```python
from build123d import *

# Parameters (mm, degrees)
BOX085026_W          = 9
BOX085026_H          = 1
BOX085026_DEPTH      = 3.85
FILLET005011017017_R = 0.49
BOX085027_W          = 9
BOX085027_H          = 1
BOX085027_DEPTH      = 3.85
FILLET005011017018_R = 0.49
BOX085028_W          = 9
BOX085028_H          = 1
BOX085028_DEPTH      = 3.85
FILLET005011017019_R = 0.49
BOX085029_W          = 9
BOX085029_H          = 1
BOX085029_DEPTH      = 3.85
FILLET005011017020_R = 0.49
BOX085030_W          = 9
BOX085030_H          = 1
BOX085030_DEPTH      = 3.85
FILLET005011017021_R = 0.49
BOX085025_W          = 9
BOX085025_H          = 9
BOX085025_DEPTH      = 1.7


with BuildPart() as fillet005011017017:
    # Box085026 → Box085026 (new body)
    with BuildSketch(Plane(origin=(25.897, 21.115, 10), x_dir=(1, 0, 0), z_dir=(0, 0, 1))):
        with Locations((4.5, 0.5)):
            Rectangle(BOX085026_W, BOX085026_H)
    extrude(amount=BOX085026_DEPTH)

    # Fillet005011017017
    fillet005011017017_edges = [fillet005011017017.edges().sort_by_distance(p)[0] for p in [
        (30.397, 21.115, 13.85),
        (30.397, 22.115, 13.85),
    ]]
    fillet(fillet005011017017_edges, radius=FILLET005011017017_R)


with BuildPart() as fillet005011017018:
    # Box085027 → Box085027 (new body)
    with BuildSketch(Plane(origin=(25.897, 21.115, 10), x_dir=(1, 0, 0), z_dir=(0, 0, 1))):
        with Locations((4.5, 0.5)):
            Rectangle(BOX085027_W, BOX085027_H)
    extrude(amount=BOX085027_DEPTH)

    # Fillet005011017018
    fillet005011017018_edges = [fillet005011017018.edges().sort_by_distance(p)[0] for p in [
        (30.397, 21.115, 13.85),
        (30.397, 22.115, 13.85),
    ]]
    fillet(fillet005011017018_edges, radius=FILLET005011017018_R)


with BuildPart() as fillet005011017018_1:
    # Fillet005011017018 placement: moved
    add(fillet005011017018.part.moved(Location((0, 2, 0))))


with BuildPart() as fillet005011017019:
    # Box085028 → Box085028 (new body)
    with BuildSketch(Plane(origin=(25.897, 21.115, 10), x_dir=(1, 0, 0), z_dir=(0, 0, 1))):
        with Locations((4.5, 0.5)):
            Rectangle(BOX085028_W, BOX085028_H)
    extrude(amount=BOX085028_DEPTH)

    # Fillet005011017019
    fillet005011017019_edges = [fillet005011017019.edges().sort_by_distance(p)[0] for p in [
        (30.397, 21.115, 13.85),
        (30.397, 22.115, 13.85),
    ]]
    fillet(fillet005011017019_edges, radius=FILLET005011017019_R)


with BuildPart() as fillet005011017019_1:
    # Fillet005011017019 placement: moved
    add(fillet005011017019.part.moved(Location((0, 4, 0))))


with BuildPart() as fillet005011017020:
    # Box085029 → Box085029 (new body)
    with BuildSketch(Plane(origin=(25.897, 21.115, 10), x_dir=(1, 0, 0), z_dir=(0, 0, 1))):
        with Locations((4.5, 0.5)):
            Rectangle(BOX085029_W, BOX085029_H)
    extrude(amount=BOX085029_DEPTH)

    # Fillet005011017020
    fillet005011017020_edges = [fillet005011017020.edges().sort_by_distance(p)[0] for p in [
        (30.397, 21.115, 13.85),
        (30.397, 22.115, 13.85),
    ]]
    fillet(fillet005011017020_edges, radius=FILLET005011017020_R)


with BuildPart() as fillet005011017020_1:
    # Fillet005011017020 placement: moved
    add(fillet005011017020.part.moved(Location((0, 6, 0))))


with BuildPart() as fillet005011017021:
    # Box085030 → Box085030 (new body)
    with BuildSketch(Plane(origin=(25.897, 21.115, 10), x_dir=(1, 0, 0), z_dir=(0, 0, 1))):
        with Locations((4.5, 0.5)):
            Rectangle(BOX085030_W, BOX085030_H)
    extrude(amount=BOX085030_DEPTH)

    # Fillet005011017021
    fillet005011017021_edges = [fillet005011017021.edges().sort_by_distance(p)[0] for p in [
        (30.397, 21.115, 13.85),
        (30.397, 22.115, 13.85),
    ]]
    fillet(fillet005011017021_edges, radius=FILLET005011017021_R)


with BuildPart() as fillet005011017021_1:
    # Fillet005011017021 placement: moved
    add(fillet005011017021.part.moved(Location((0, 8, 0))))


with BuildPart() as obj1:
    # Box085025 → Box085025 (new body)
    with BuildSketch(Plane(origin=(25.897, 21.115, 8.3), x_dir=(1, 0, 0), z_dir=(0, 0, 1))):
        with Locations((4.5, 4.5)):
            Rectangle(BOX085025_W, BOX085025_H)
    extrude(amount=BOX085025_DEPTH)

    # Fusion004008002002002001007002002014: union Fillet005011017017, Fillet005011017018, Fillet005011017019, Fillet005011017020, Fillet005011017021
    add(fillet005011017017.part)
    add(fillet005011017018_1.part)
    add(fillet005011017019_1.part)
    add(fillet005011017020_1.part)
    add(fillet005011017021_1.part)


with BuildPart() as obj1_1:
    # Fusion004008002002002001007002002014 placement: moved
    add(obj1.part.moved(Location((0, 0, -1))))


solid = obj1_1.part
```
Geometry check sheet. Reference: the model listing, model coordinates, mm. A direction names the side the tool comes from. Give positions to 0.01 mm unless a question says otherwise; leave off trailing zeros. Loops run counter-clockwise (first coordinate to the right, second up) from the corner with the lowest first, then second, coordinate; pieces in that order, holes last. Notation, with made-up numbers: M 4,-3.5 L 58,-3.5 A17 ccw 58,2.5 Z; hole C 9,-24 d10. An arc over 180 degrees is marked long. Write item = value, one per line. Start each with the question number.
1. Draft check along Y on faces 3 (the face through (30.3, 24.6, 9)), 4 (the face through (34.897, 25.6, 9.4)), 5 (the face through (30, 21.115, 10)). Enter one of: +Y half, -Y half, draft (parallel to the pull), parting line (faces both ways), or undercut.
2. Section check C-C, the plane y = 29.25. Enter the section's corners in (x, z).
3. Section check A-A, the plane z = 10. Enter the section's corners in (x, y) (3 decimals), plus the area to 3 significant figures.
4. Go/stop test with flat-tipped pins: P1, Ø0.5, axis at x = 32.5, y = 29, coming from the +Z side; P2, Ø1.1, axis at x = 28.5, y = 27, coming from the +Z side; P3, Ø0.5, axis at x = 31.5, y = 24.5, coming from the +Z side. Record where each tip stops, or that it passes through.
5. Section check D-D, the plane y = 26. Enter the section's corners in (x, z).
6. Thickness scan on probe 1 along Y at (x, z) = (26.75, 9.9) (3 decimals); probe 2 along Y at (x, z) = (29.25, 12.65); probe 3 along Z at (x, y) = (31.25, 27). Record the ranges inside material, lowest first.
7. Tool access check on faces 1 (the face through (30, 24.115, 11)), 2 (the face through (25.897, 25.6, 9.4)). Record the directions out of +Z, -Z, +X, -X, +Y, -Y that give a thin tool (end or side, any length) a straight path to the whole face; none if there is none.
Values follow:
q1.face_3 = undercut
q1.face_4 = draft
q1.face_5 = -Y half
q2.outline = M 25.9,7.3 L 34.9,7.3 L 34.9,12.7 L 25.9,12.7 Z
q3.outline = M 25.897,21.115 L 34.897,21.115 L 34.897,22.115 L 25.897,22.115 Z; M 25.897,23.115 L 34.897,23.115 L 34.897,24.115 L 25.897,24.115 Z; M 25.897,25.115 L 34.897,25.115 L 34.897,26.115 L 25.897,26.115 Z; M 25.897,27.115 L 34.897,27.115 L 34.897,28.115 L 25.897,28.115 Z; M 25.897,29.115 L 34.897,29.115 L 34.897,30.115 L 25.897,30.115 Z
q3.area = 45.0 mm^2
q4.P1 = 12.7
q4.P2 = 12.85
q4.P3 = 9
q5.outline = M 25.9,7.3 L 34.9,7.3 L 34.9,12.68 L 25.9,12.68 Z
q6.probe_1 = 21.115 to 22.115, 23.115 to 24.115, 25.115 to 26.115, 27.115 to 28.115, 29.115 to 30.115
q6.probe_2 = 21.21 to 22.02, 23.21 to 24.02, 25.21 to 26.02, 27.21 to 28.02, 29.21 to 30.02
q6.probe_3 = 7.3 to 9
q7.face_1 = +Z, +X, -X
q7.face_2 = +Z, -Z, -X, +Y, -Y
